Drawing for the job (mm, zero at the part's lowest x, y, z). A direction names the side the tool comes from. Coordinates: 2 decimals unless noted, no trailing zeros. Order: outer loops, then holes, each group sorted by start corner. A loop starts at its lowest first (then second) coordinate and runs counter-clockwise, first axis right, second up.
1) Wall check: L1, parallel to X at y = 33, z = 7.62; L2, parallel to Y at x = 19.05, z = 4.25; L3, parallel to X at y = 6, z = 9. Give the ranges that are in metal, low to high.
2) Cut at A-A (y = 19.05). List the corners of the cut face in (x, z) (1 decimal), and give its area (3 significant figures).
3) Mould opens along X. For the marked faces 1, 2 and 3 say: +X half, -X half, draft (parallel to the pull), parting line (faces both ways), or undercut.
4) Cut at D-D (y = 5.5). List the corners of the cut face in (x, z) (3 decimals).
5) Pin check, flat tips, straight feed: pin 1 Ø3 at (x, z) = (9.525, 7.62) entering from -Y; pin 2 Ø3 at (x, z) = (17, 25.5) entering from -Y; pin 3 Ø1.6 at (x, y) = (19, 19) entering from -Z. Stop position of each tip, or through.
6) Tool access for the marked faces 4, 5, 6, 7 and 8: list every direction of +Z, -Z, +X, -X, +Y, -Y with a clear straight run to the whole face (end or side of a thin tool).
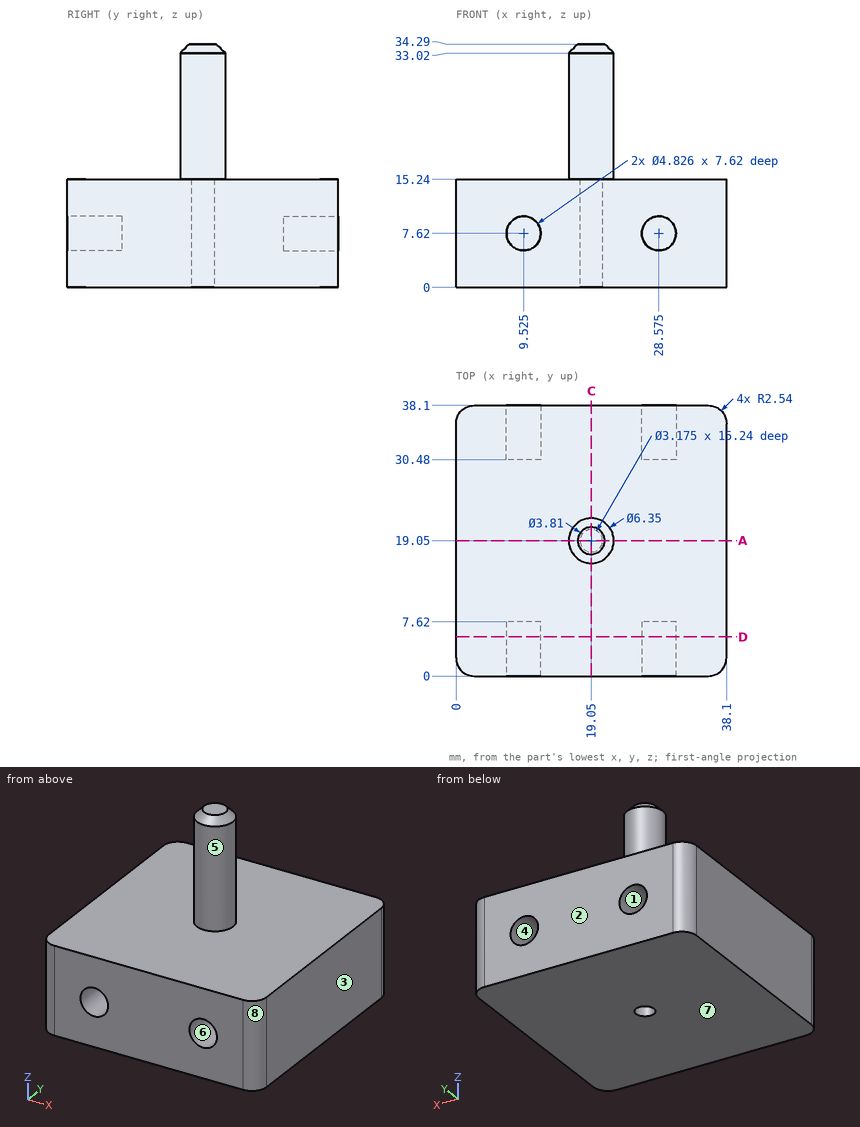
Geometry check:
1. L1: x = 0 to 7.11, 11.94 to 26.16, 30.99 to 38.1
1. L2: y = 0 to 17.46, 20.64 to 38.1
1. L3: x = 0 to 7.55, 11.5 to 26.6, 30.55 to 38.1
2. outline: (0, 0) - (17.5, 0) - (17.5, 15.2) - (20.6, 15.2) - (20.6, 0) - (38.1, 0) - (38.1, 15.2) - (22.2, 15.2) - (22.2, 33) - (21, 34.3) - (17.1, 34.3) - (15.9, 33) - (15.9, 15.2) - (0, 15.2) - close
2. area: 652 mm2
3. face 1: undercut
3. face 2: draft
3. face 3: +X half
4. outline: (0, 0) - (38.1, 0) - (38.1, 15.24) - (0, 15.24) - close; hole circle Ø4.826 at (9.525, 7.62); hole circle Ø4.826 at (28.575, 7.62)
5. pin 1: stops at y = 7.62
5. pin 2: stops at y = 15.92
5. pin 3: stops at z = 15.24
6. face 4: +Y
6. face 5: +Z
6. face 6: -Y
6. face 7: -Z, +X, -X, +Y, -Y
6. face 8: +Z, -Z, +X, -Y
